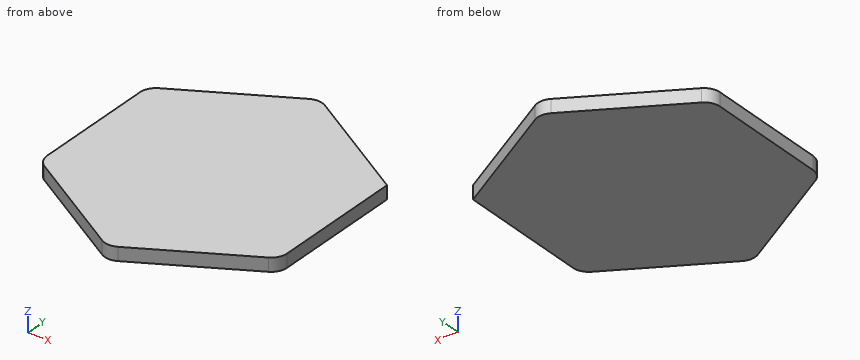
```python
from build123d import *

# Parameters (mm, degrees)
F1_DEPTH = 5


with BuildPart() as f1:
    # F0 (on Top) → F1 (new body)
    with BuildSketch(Plane.XY):
        with BuildLine():
            Line((45, 25.980762), (3, 50.229473))
            ThreePointArc((3, 50.229473), (0, 51.033321), (-3, 50.229473))
            Line((-3, 50.229473), (-42, 27.712813))
            ThreePointArc((-42, 27.712813), (-44.196152, 25.51666), (-45, 22.51666))
            Line((-45, 22.51666), (-45, -22.51666))
            ThreePointArc((-45, -22.51666), (-44.196152, -25.51666), (-42, -27.712813))
            Line((-42, -27.712813), (-3, -50.229473))
            ThreePointArc((-3, -50.229473), (0, -51.033321), (3, -50.229473))
            Line((3, -50.229473), (42, -27.712813))
            ThreePointArc((42, -27.712813), (44.196152, -25.51666), (45, -22.51666))
            Line((45, -22.51666), (45, 25.980762))
        make_face()
    extrude(amount=F1_DEPTH)


solid = f1.part
```
Here's how the part is built. I have some questions about the finished solid (model axes, mm). Coordinates: 2 decimals unless noted, no trailing zeros. Order: outer loops, then holes, each group sorted by start corner. A loop starts at its lowest first (then second) coordinate and runs counter-clockwise, first axis right, second up.
1) Imagine slicing it at B-B on x = 6.5. List the corners of the cut face in (y, z) for me, and give its area (3 significant figures).
2) Will this pin go through, and if not, where does the flat tip stop? pin 1 (3 mm diameter, centred on x = -22, z = 1.5, fed in from +Y).
3) Imagine slicing it at C-C on y = -30. List the corners of the cut face in (x, z) for me, and give its area (3 significant figures).
4) I need wall thicknesses on line 1 (X direction, y = 31.5, z = 1.65); line 2 (X direction, y = -28.5, z = 1.6); line 3 (Y direction, x = -38.5, z = 4.5). Which ranges of each line are inside material? Lowest first, please.
5) Imagine slicing it at A-A on z = 3.9. List the corners of the cut face in (x, y) for me, and give its area (3 significant figures).
Response values:
1. outline: (-48.21, 0) - (48.21, 0) - (48.21, 5) - (-48.21, 5) - close
1. area: 482 mm2
2. pin 1: stops at y = 40.13
3. outline: (-38.04, 0) - (38.04, 0) - (38.04, 5) - (-38.04, 5) - close
3. area: 380 mm2
4. line 1: x = -35.44 to 35.44
4. line 2: x = -40.64 to 40.64
4. line 3: y = -29.73 to 29.73
5. outline: (-45, -22.52) arc R6 ccw to (-42, -27.71) - (-3, -50.23) arc R6 ccw to (3, -50.23) - (42, -27.71) arc R6 ccw to (45, -22.52) - (45, 25.98) - (3, 50.23) arc R6 ccw to (-3, 50.23) - (-42, 27.71) arc R6 ccw to (-45, 22.52) - close
5. area: 7,010 mm2
